Source: three-view drawing plus pictorial views. Frame: mm from the lowest corner of the part. A direction names the side the tool comes from. Give positions to 0.01 mm unless a question says otherwise; leave off trailing zeros. Write each loop counter-clockwise with the first axis right and the second up, starting at its lowest first coordinate (ties: lowest second). Pieces come first, ordered by that corner, then holes. Notation, with made-up numbers: M -35.75,28 L -14.75,28 A26 ccw -14.75,60 Z; hole C -3,83.25 d10. An arc over 180 degrees is marked long. Return JSON: item names as keys, results as strings.
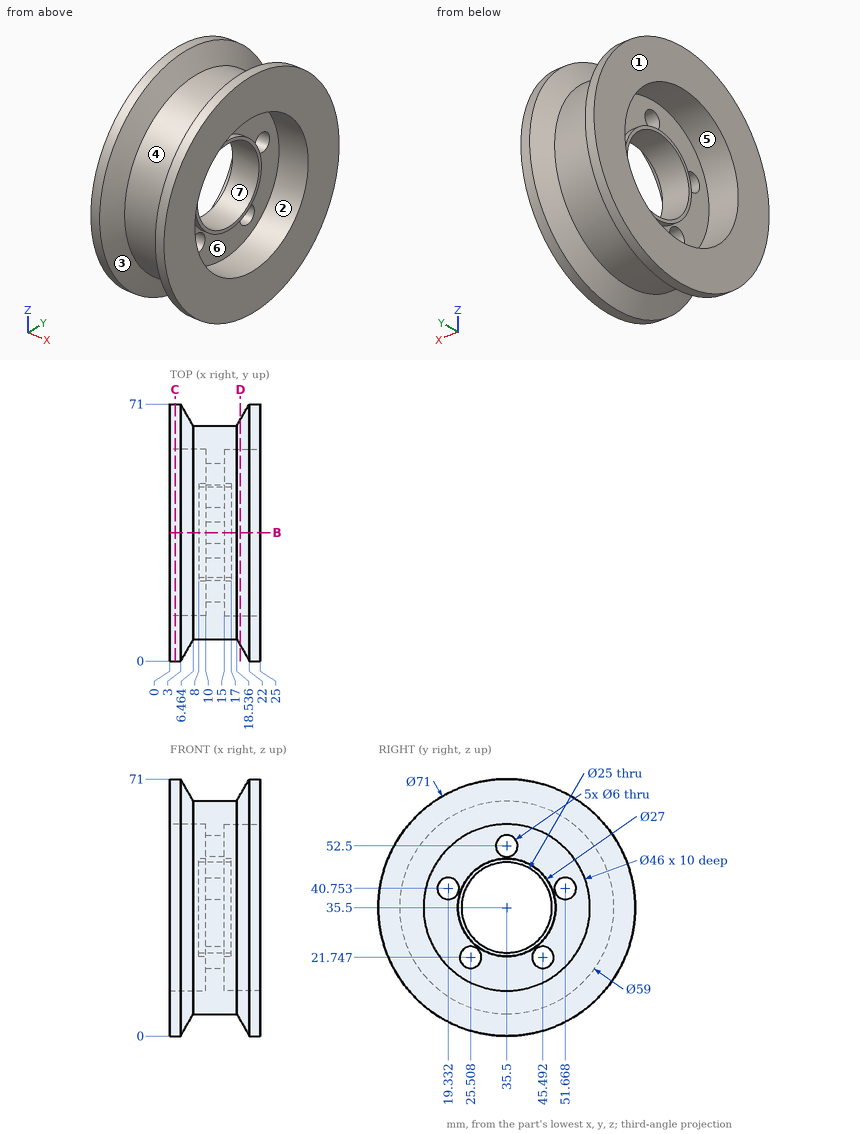
1) Cut plane B-B, the plane y = 35.5. Give the number of separate pieces and of enclosed holes in the cut face.
Numbers:
{"separate pieces": "3", "enclosed holes": "0"}
2) Cut plane D-D, the plane x = 19.5. Return the cut outline in (y, z).
Numbers:
{"outline": "C 35.5,35.5 d62.34; hole C 35.5,35.5 d46"}
3) Cut plane C-C, the plane x = 1.5. Return the cut outline in (y, z), then the cut area to 3 significant figures.
Numbers:
{"outline": "C 35.5,35.5 d71; hole C 35.5,35.5 d46", "area": "2,300 mm²"}
4) Line query: line 1 (Y direction, x = 13.5, z = 41) (1 decimal); line 2 (Z direction, x = 9.25, y = 38.5) (1 decimal); line 3 (Y direction, x = 6.5, z = 35.5). Output: solid intervals per line, ascending. Write a range as [from, to].
Numbers:
{"line 1": "y = [6.5, 16.3], [22.3, 24.3], [46.7, 48.7], [54.7, 64.5]", "line 2": "z = [6.2, 12.7], [22.3, 23.4], [47.6, 48.7], [58.3, 64.8]", "line 3": "y = [6, 12.5], [58.5, 65]"}
5) Set-up query: the marked faces 4, 5, 6 and 7. Return all of +Z, -Z, +X, -X, +Y, -Y with unobstructed straight access to the full face (end or side cutting, diameter ignored); none if empty.
Numbers:
{"face 4": "none", "face 5": "-X", "face 6": "+X", "face 7": "+X, -X"}
6) Draft query along Z for the marked faces 1, 2 and 3. Return one class per face: released by +Z, released by -Z, zero draft, split by the parting line, or undercut.
Numbers:
{"face 1": "zero draft", "face 2": "undercut", "face 3": "split by the parting line"}
7) Contact query for flat-ended pins moving along their axis: pin 1 Ø2 at (x, y) = (18.5, 49) entering from +Z (1 decimal); pin 2 Ø9.5 at (y, z) = (51.67, 40.75) entering from -X; pin 3 Ø2 at (y, z) = (61.5, 14) entering from -X; pin 4 Ø10 at (x, y) = (10, 18.5) entering from -Z (1 decimal). Output: stop coordinate, or through.
Numbers:
{"pin 1": "stops at z = 63.7", "pin 2": "stops at x = 8", "pin 3": "stops at x = 0", "pin 4": "stops at z = 7.9"}
